Work out the finished part from the listing and answer in its coordinate system (mm). Face numbers are marked on the shaded views. Round coordinates to 2 decimals unless told otherwise and drop trailing zeros. Order: outer loops, then holes, each group sorted by start corner. A loop starts at its lowest first (then second) coordinate and runs counter-clockwise, first axis right, second up. Notation, with made-up numbers: M -19.5,41.5 L 15.5,41.5 A26 ccw 15.5,61.5 Z; hole C 87.25,72.25 d6. An arc over 180 degrees is marked long. Return JSON: item names as keys, results as strings.
from build123d import *

# Parameters (mm, degrees)
SKETCH_2_R               = 25
SKETCH_2_R_2             = 21
EXTRUDE_2_DEPTH          = 122
CUT_EXTRUDE_2_DEPTH      = 10
CUT_EXTRUDE_2_DEPTH_BACK = 135.197615478
SKETCH_4_R               = 2


with BuildPart() as part:
    # Sketch 2 → Extrude 2 (new body)
    with BuildSketch(Plane(origin=(0, 0, 0), x_dir=(0, 0, -1), z_dir=(1, 0, 0))):
        with Locations(Location((0, 0, 0), (0, 0, 180))):
            Circle(SKETCH_2_R)
        with Locations(Location((0, 0, 0), (0, 0, 180))):
            Circle(SKETCH_2_R_2, mode=Mode.SUBTRACT)
    extrude(amount=EXTRUDE_2_DEPTH)

    # Sketch 4 → Cut-Extrude 2 (cut, two sides: drawn at the far end of the back side and taken through both)
    with BuildSketch(Plane.XY.offset(25).offset(-CUT_EXTRUDE_2_DEPTH_BACK)):
        with Locations(Location((12.5, 0, 0), (0, 0, 180))):
            Circle(SKETCH_4_R)
        with Locations(Location((109.5, 0, 0), (0, 0, 180))):
            Circle(SKETCH_4_R)
        with Locations(Location((25, 0, 0), (0, 0, 180))):
            Circle(SKETCH_4_R)
        with Locations(Location((37.5, 0, 0), (0, 0, 180))):
            Circle(SKETCH_4_R)
        with Locations(Location((97, 0, 0), (0, 0, 180))):
            Circle(SKETCH_4_R)
        with Locations(Location((84.5, 0, 0), (0, 0, 180))):
            Circle(SKETCH_4_R)
    extrude(amount=CUT_EXTRUDE_2_DEPTH + CUT_EXTRUDE_2_DEPTH_BACK, mode=Mode.SUBTRACT)


solid = part.part
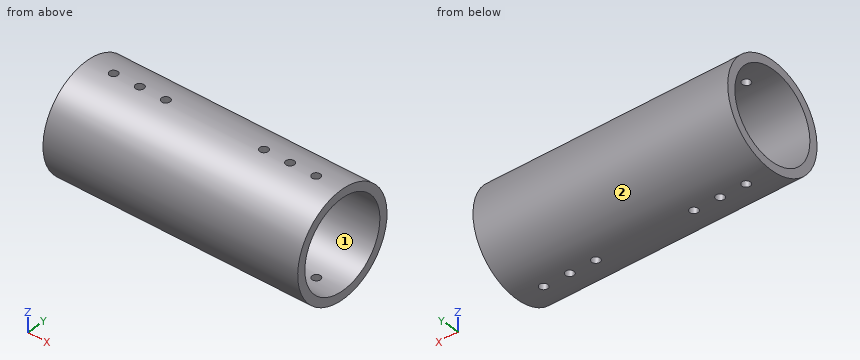
Item 1: Consider line 1 along Y through (x, z) = (65, 17); line 2 along Y through (x, z) = (67.5, -5.5); line 3 along Z through (x, y) = (69, 5). Determine where each line is inside the solid, lowest interval first. Write a range as [from, to].
Output:
{"line 1": "y = [-18.33, -12.33], [12.33, 18.33]", "line 2": "y = [-24.39, -20.27], [20.27, 24.39]", "line 3": "z = [-24.49, -20.4], [20.4, 24.49]"}
Item 2: Find section B-B (x = 109.5). Determine the outline of the cut face in (y, z), plus the area to 3 significant figures.
Output:
{"outline": "M -2,-24.92 L -2,-20.9 A21 cw -2,20.9 L -2,24.92 A25 ccw Z; M 2,-24.92 A25 ccw 2,24.92 L 2,20.9 A21 cw 2,-20.9 Z", "area": "546 mm^2"}
Item 3: The mould has two halves that part along Z. Classify the marked faces 1 and 2: pulls with the +Z half, pulls with the -Z half, needs draft (parallel to the pull), parting line crosses it, or undercut.
Output:
{"face 1": "undercut", "face 2": "parting line crosses it"}
Item 4: Find section D-D (x = 73.5). Determine the outline of the cut face in (y, z).
Output:
{"outline": "C 0,0 d50; hole C 0,0 d42"}
Item 5: Find section C-C (y = 0). State how many separate pieces and enclosed holes the cut face has, plus the area to 3 significant figures.
Output:
{"separate pieces": "14", "enclosed holes": "0", "area": "784 mm^2"}
Item 6: Each of these flat-tipped pins is pushed along its axis until it touches: pin 1 (3 mm diameter, centred on x = 97, y = 0, fed in from -Z); pin 2 (6 mm diameter, centred on x = 43.5, z = -19.5, fed in from +Y); pin 3 (5 mm diameter, centred on x = 76, y = 12.5, fed in from +Z); pin 4 (1.5 mm diameter, centred on x = 37, y = -18, fed in from +Z). Where does it stop, or does it pass through?
Output:
{"pin 1": "passes through", "pin 2": "stops at y = 18.78", "pin 3": "stops at z = 22.91", "pin 4": "stops at z = 18.1"}
Item 7: Find section A-A (z = 0). Determine the outline of the cut face in (x, y), plus the area to 3 significant figures.
Output:
{"outline": "M 0,-25 L 122,-25 L 122,-21 L 0,-21 Z; M 0,21 L 122,21 L 122,25 L 0,25 Z", "area": "976 mm^2"}
